The drawing under review shows one solid part. Ordinate dimensions are in mm from its lowest x, y, z. A direction names the side the tool comes from. Give positions to 0.01 mm unless a question says otherwise; leave off trailing zeros. Order: outer loops, then holes, each group sorted by start corner. A loop starts at its lowest first (then second) coordinate and runs counter-clockwise, first axis right, second up. Notation, with made-up numbers: (48.5, -7) - (103.5, -7) arc R31 ccw to (103.5, 27) - close; hole circle Ø4 at (4, 11.5). An arc over 180 degrees is marked (long way). Use CSV: the item, a comma, the result in double quotes. Start each with the question number.
1. To check wall thickness, follow line 1 (Z direction, x = 24, y = 4.55); line 2 (X direction, y = 3.1, z = 2.25); line 3 (Y direction, x = 12, z = 25.75). State the ranges of each line that lie inside material, in increasing order. Write a range as [from, to].
2. For pin 1 (3 mm diameter, centred on x = 3, z = 24, fed in from +Y); pin 2 (2 mm diameter, centred on x = 23.5, z = 19, fed in from -Y), all flat-tipped, find the tip position at first contact; note any pin that passes through.
3. Machinability: for the marked faces 4 and 5, which of the approach directions +Z, -Z, +X, -X, +Y, -Y give a long, thin tool a straight path to every point of the face, cutting with its end or side? Answer none if there is none.
4. Take a section at B-B, the plane z = 24. State the section outline as (x, y) points, then the cut area to 3 significant figures.
5. Take a section at D-D, the plane z = 13.5. State the section outline as (x, y) points, then the cut area to 3 significant figures.
6. Take a section at C-C, the plane y = 4.55. State the section outline as (x, z) points.
7. Draft analysis for pull direction X (two halves, no side actions). For the marked faces 1, 2 and 3, state which applies: released by +X, released by -X, zero draft, split by the parting line, or undercut.
8. Take a section at A-A, the plane x = 3. State the section outline as (y, z) points, then the cut area to 3 significant figures.
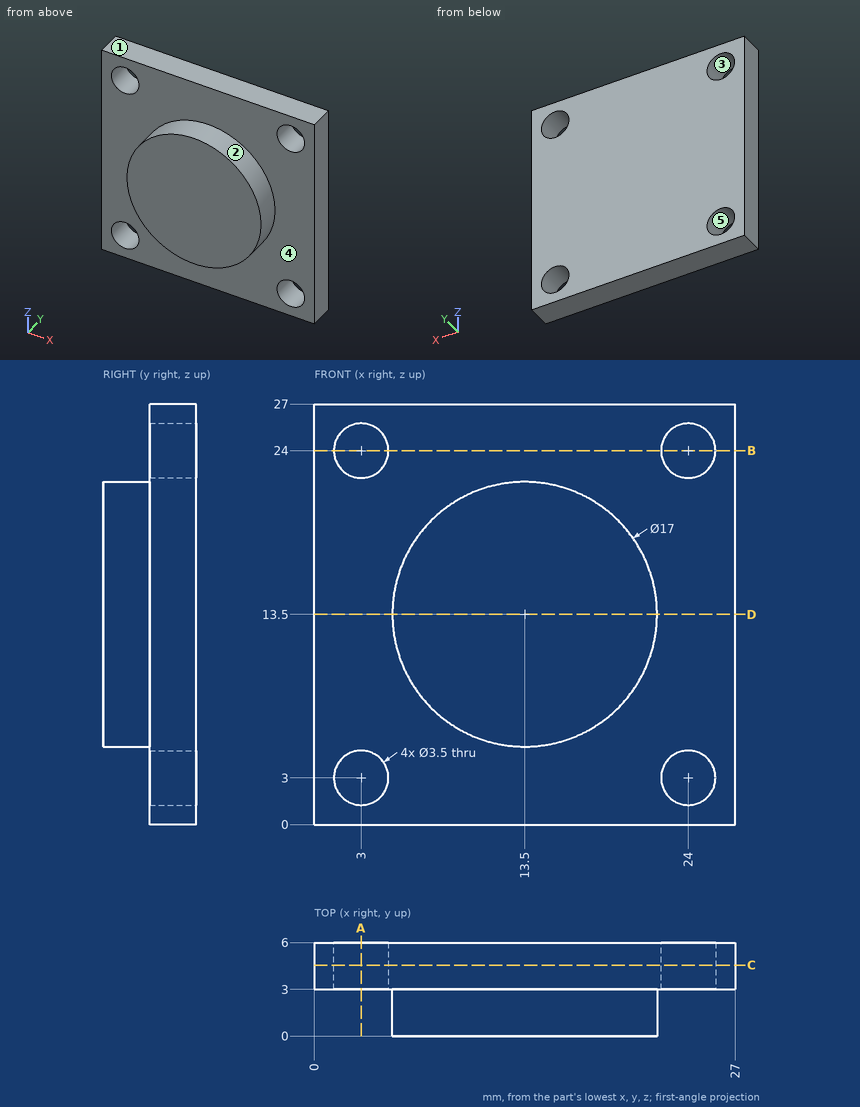
Determined:
1,line 1,"z = [0, 1.25], [4.75, 22.25], [25.75, 27]"
1,line 2,"x = [0, 1.42], [4.58, 22.42], [25.58, 27]"
1,line 3,"y = [3, 6]"
2,pin 1,"passes through"
2,pin 2,"stops at y = 3"
3,face 4,"-Y"
3,face 5,"+Y, -Y"
4,outline,"(0, 3) - (1.25, 3) - (1.25, 6) - (0, 6) - close; (4.75, 3) - (22.25, 3) - (22.25, 6) - (4.75, 6) - close; (25.75, 3) - (27, 3) - (27, 6) - (25.75, 6) - close"
4,area,"60.0 mm²"
5,outline,"(0, 3) - (5, 3) - (5, 0) - (22, 0) - (22, 3) - (27, 3) - (27, 6) - (0, 6) - close"
5,area,"132 mm²"
6,outline,"(0, 0) - (27, 0) - (27, 27) - (0, 27) - close; hole circle Ø3.5 at (3, 3); hole circle Ø3.5 at (3, 24); hole circle Ø3.5 at (24, 3); hole circle Ø3.5 at (24, 24)"
7,face 1,"zero draft"
7,face 2,"split by the parting line"
7,face 3,"undercut"
8,outline,"(3, 0) - (6, 0) - (6, 1.25) - (3, 1.25) - close; (3, 4.75) - (6, 4.75) - (6, 22.25) - (3, 22.25) - close; (3, 25.75) - (6, 25.75) - (6, 27) - (3, 27) - close"
8,area,"60.0 mm²"
